Model file for the job. Use its own axes, mm. A direction names the side the tool comes from. Round coordinates to 2 decimals unless told otherwise and drop trailing zeros. Order: outer loops, then holes, each group sorted by start corner. A loop starts at its lowest first (then second) coordinate and runs counter-clockwise, first axis right, second up. Notation, with made-up numbers: (88, -38) -> (120, -38) arc R27 ccw to (120, -15) -> close; hole circle Ø8 at (20, 56.5). An arc over 180 degrees is marked (long way). Answer as CSV lines item,"result".
```python
from build123d import *

# Parameters (mm, degrees)
SKETCH2_W           = 267.6500108
SKETCH2_H           = 83.5000108
BOSS_EXTRUDE2_DEPTH = 10
SKETCH3_W           = 267.6500108
SKETCH3_H           = 83.5000108
SKETCH3_W_2         = 247.7440108
SKETCH3_H_2         = 63.5000108
BOSS_EXTRUDE3_DEPTH = 38.1


with BuildPart() as part:
    # Sketch2 → Boss-Extrude2 (new body)
    with BuildSketch(Plane(origin=(0, 0, 0), x_dir=(1, 0, 0), z_dir=(0, 1, 0))):
        Rectangle(SKETCH2_W, SKETCH2_H)
    extrude(amount=BOSS_EXTRUDE2_DEPTH)

    # Sketch3 → Boss-Extrude3 (add)
    with BuildSketch(Plane(origin=(0, 10, 0), x_dir=(1, 0, 0), z_dir=(0, 1, 0))):
        Rectangle(SKETCH3_W, SKETCH3_H)
        with Locations((0.047, 0)):
            Rectangle(SKETCH3_W_2, SKETCH3_H_2, mode=Mode.SUBTRACT)
    extrude(amount=BOSS_EXTRUDE3_DEPTH)


solid = part.part
```
Q1. Wall check: L1, parallel to X at y = 18, z = 11 (3 decimals); L2, parallel to Z at x = -2.5, y = 19; L3, parallel to Y at x = -38, z = -21.5. Give the ranges that are in metal, low to high. Write a range as [from, to].
Checks:
L1,"[-133.825, -123.825], [123.919, 133.825]"
L2,"[-41.75, -31.75], [31.75, 41.75]"
L3,"[0, 10]"
Q2. Saw through at A-A (z = -18.5). Write the cut outline in (x, y) (3 decimals), plus the area to 3 significant figures.
Checks:
outline,"(-133.825, 0) -> (133.825, 0) -> (133.825, 48.1) -> (123.919, 48.1) -> (123.919, 10) -> (-123.825, 10) -> (-123.825, 48.1) -> (-133.825, 48.1) -> close"
area,"3,430 mm²"
Q3. Saw through at B-B (y = 32.5). Write the cut outline in (x, z) (3 decimals), plus the area to 3 significant figures.
Checks:
outline,"(-133.825, -41.75) -> (133.825, -41.75) -> (133.825, 41.75) -> (-133.825, 41.75) -> close; hole (-123.825, -31.75) -> (123.919, -31.75) -> (123.919, 31.75) -> (-123.825, 31.75) -> close"
area,"6,620 mm²"
Q4. Tool access for faces 4 (the flat face through (-2, 29, 31.75)), 5 (the flat face through (-2, 0, -1)): list every direction of +Z, -Z, +X, -X, +Y, -Y with a clear straight run to the whole face (end or side of a thin tool).
Checks:
face 4,"+Y"
face 5,"+Z, -Z, +X, -X, -Y"
Q5. Mould opens along X. For faces 1 (the flat face through (133.825, 24, 1)), 2 (the flat face through (-123.825, 29, 0)), 3 (the flat face through (-11, 48.1, 34)) say: +X half, -X half, draft (parallel to the pull), parting line (faces both ways), or undercut.
Checks:
face 1,"+X half"
face 2,"undercut"
face 3,"draft"
Q6. Saw through at C-C (x = -94). Write the cut outline in (y, z), plus the area to 3 significant figures.
Checks:
outline,"(0, -41.75) -> (48.1, -41.75) -> (48.1, -31.75) -> (10, -31.75) -> (10, 31.75) -> (48.1, 31.75) -> (48.1, 41.75) -> (0, 41.75) -> close"
area,"1,600 mm²"
Q7. Flat gauge pins, fed straight in: pin 1 (2 mm diameter, centred on x = 2, z = -30.5, fed in from -Y); pin 2 (3 mm diameter, centred on x = 103.5, z = 0, fed in from +Y). Where does each tip first touch, or does it go through?
Checks:
pin 1,"y = 0"
pin 2,"y = 10"
